from build123d import *

# Parameters (mm, degrees)
SKETCH1_R            = 4.5
SKETCH1_R_2          = 1.25
SKETCH1_R_3          = 1.75
SKETCH1_R_4          = 2.75
BOSS_EXTRUDE10_DEPTH = 5
SKETCH1_16_R         = 1.25
BOSS_EXTRUDE11_DEPTH = 5
SKETCH3_R            = 1.75
CUT_EXTRUDE5_DEPTH   = 17
CUT_EXTRUDE7_DEPTH   = 10
SKETCH1_18_R         = 4.5
SKETCH1_18_R_2       = 1.75
BOSS_EXTRUDE12_DEPTH = 5
SKETCH10_R           = 32.76798012
SKETCH10_R_2         = 29.85
BOSS_EXTRUDE13_DEPTH = 13
SKETCH11_R           = 27.095
CUT_EXTRUDE8_DEPTH   = 13
BOSS_EXTRUDE14_DEPTH = 3
SKETCH13_W           = 12
SKETCH13_H           = 4
BOSS_EXTRUDE15_DEPTH = 25
SKETCH14_R           = 1.25
CUT_EXTRUDE9_DEPTH   = 25
FILLET1_R            = 2.5
SKETCH18_W           = 172.850535033
SKETCH18_H           = 5
BOSS_EXTRUDE18_DEPTH = 18
SKETCH19_W           = 18
SKETCH19_H           = 172.850535033
BOSS_EXTRUDE19_DEPTH = 22
SKETCH20_R           = 7.5
CUT_EXTRUDE11_DEPTH  = 208
FILLET3_R            = 10


with BuildPart() as part:
    # Sketch1 → Boss-Extrude10 (new body)
    with BuildSketch(Plane(origin=(0, 0, 0), x_dir=(1, 0, 0), z_dir=(0, 1, 0))):
        with BuildLine():
            Line((-32.774, -22.380453712), (-32.774, 177.619546288))
            ThreePointArc((-32.774, 177.619546288), (0, 210.393546288), (32.774, 177.619546288))
            Line((32.774, 177.619546288), (32.774, -22.380453712))
            ThreePointArc((32.774, -22.380453712), (0, -55.154453712), (-32.774, -22.380453712))
        make_face()
        with Locations(Location((0, 177.619546288, 0), (0, 0, 270))):
            Circle(SKETCH1_R, mode=Mode.SUBTRACT)
        with Locations(Location((-6.733414, 37.119546288, 0), (0, 0, 270))):
            Circle(SKETCH1_R_2, mode=Mode.SUBTRACT)
        with Locations(Location((-6.733414, 27.619546288, 0), (0, 0, 270))):
            Circle(SKETCH1_R_2, mode=Mode.SUBTRACT)
        with Locations(Location((0, 53.605186475, 0), (0, 0, 270))):
            Circle(SKETCH1_R_3, mode=Mode.SUBTRACT)
        with Locations(Location((-14.032659813, 67.637846288, 0), (0, 0, 270))):
            Circle(SKETCH1_R_3, mode=Mode.SUBTRACT)
        with Locations(Location((0, 81.6705061, 0), (0, 0, 270))):
            Circle(SKETCH1_R_3, mode=Mode.SUBTRACT)
        with Locations(Location((14.032659813, 67.637846288, 0), (0, 0, 270))):
            Circle(SKETCH1_R_3, mode=Mode.SUBTRACT)
        with Locations(Location((0, 67.637846288, 0), (0, 0, 270))):
            Circle(SKETCH1_R, mode=Mode.SUBTRACT)
        with Locations(Location((0, -9.380453712, 0), (0, 0, 270))):
            Circle(SKETCH1_R_4, mode=Mode.SUBTRACT)
        with Locations(Location((11.258330249, -15.880453712, 0), (0, 0, 270))):
            Circle(SKETCH1_R_4, mode=Mode.SUBTRACT)
        with Locations(Location((11.258330249, -28.880453712, 0), (0, 0, 270))):
            Circle(SKETCH1_R_4, mode=Mode.SUBTRACT)
        with Locations(Location((0, -35.380453712, 0), (0, 0, 270))):
            Circle(SKETCH1_R_4, mode=Mode.SUBTRACT)
        with Locations(Location((-11.258330249, -28.880453712, 0), (0, 0, 270))):
            Circle(SKETCH1_R_4, mode=Mode.SUBTRACT)
        with Locations(Location((-11.258330249, -15.880453712, 0), (0, 0, 270))):
            Circle(SKETCH1_R_4, mode=Mode.SUBTRACT)
    extrude(amount=-BOSS_EXTRUDE10_DEPTH)

    # Sketch1_16 → Boss-Extrude11 (add)
    with BuildSketch(Plane(origin=(0, 0, 0), x_dir=(1, 0, 0), z_dir=(0, 1, 0))):
        with Locations((-6.733414, 37.119546288)):
            Circle(SKETCH1_16_R)
        with Locations((-6.733414, 27.619546288)):
            Circle(SKETCH1_16_R)
    extrude(amount=-BOSS_EXTRUDE11_DEPTH)

    # Sketch3 → Cut-Extrude5 (cut)
    with BuildSketch(Plane.XZ.offset(5)):
        with Locations(Location((15, -102.056321071, 0), (0, 0, 270))):
            Circle(SKETCH3_R)
        with Locations(Location((-30.384, -67.619546288, 0), (0, 0, 270))):
            Circle(SKETCH3_R)
        with Locations(Location((-30.384, -37.619546288, 0), (0, 0, 270))):
            Circle(SKETCH3_R)
        with Locations(Location((-30.384, -97.619546288, 0), (0, 0, 270))):
            Circle(SKETCH3_R)
        with Locations(Location((-30.384, -127.619546288, 0), (0, 0, 270))):
            Circle(SKETCH3_R)
        with Locations(Location((-30.384, -157.619546288, 0), (0, 0, 270))):
            Circle(SKETCH3_R)
        with Locations(Location((30.384, -157.619546288, 0), (0, 0, 90))):
            Circle(SKETCH3_R)
        with Locations(Location((30.384, -127.619546288, 0), (0, 0, 90))):
            Circle(SKETCH3_R)
        with Locations(Location((30.384, -97.619546288, 0), (0, 0, 90))):
            Circle(SKETCH3_R)
        with Locations(Location((30.384, -67.619546288, 0), (0, 0, 90))):
            Circle(SKETCH3_R)
        with Locations(Location((30.384, -37.619546288, 0), (0, 0, 90))):
            Circle(SKETCH3_R)
    extrude(amount=-CUT_EXTRUDE5_DEPTH, mode=Mode.SUBTRACT)

    # Sketch2 → Cut-Extrude7 (cut)
    with BuildSketch(Plane.XZ):
        with BuildLine():
            Line((28, 22.380453712), (28, -4.769011255))
            Line((28, -4.769011255), (32.774000001, -4.769011255))
            Line((32.774000001, -4.769011255), (32.774000001, 22.380453712))
            ThreePointArc((32.774000001, 22.380453712), (0, 55.154453713), (-32.774000001, 22.380453712))
            Line((-32.774000001, 22.380453712), (-32.774000001, -4.769011255))
            Line((-32.774000001, -4.769011255), (-28, -4.769011255))
            Line((-28, -4.769011255), (-28, 22.380453712))
            ThreePointArc((-28, 22.380453712), (0, 50.380453712), (28, 22.380453712))
        make_face()
        with BuildLine():
            Line((-28, -4.769011255), (28, -4.769011255))
            Line((28, -4.769011255), (28, 22.380453712))
            ThreePointArc((28, 22.380453712), (0, 50.380453712), (-28, 22.380453712))
            Line((-28, 22.380453712), (-28, -4.769011255))
        make_face()
    extrude(amount=CUT_EXTRUDE7_DEPTH, mode=Mode.SUBTRACT)

    # Sketch1_18 → Boss-Extrude12 (add)
    with BuildSketch(Plane(origin=(0, 0, 0), x_dir=(1, 0, 0), z_dir=(0, 1, 0))):
        with Locations((0, 67.637846288)):
            Circle(SKETCH1_18_R)
        with Locations((14.032659813, 67.637846288)):
            Circle(SKETCH1_18_R_2)
        with Locations((0, 81.6705061)):
            Circle(SKETCH1_18_R_2)
        with Locations((0, 53.605186475)):
            Circle(SKETCH1_18_R_2)
        with Locations((-14.032659813, 67.637846288)):
            Circle(SKETCH1_18_R_2)
    extrude(amount=-BOSS_EXTRUDE12_DEPTH)

    # Sketch10 → Boss-Extrude13 (add)
    with BuildSketch(Plane.XZ.offset(5)):
        with Locations(Location((0, -177.619546288, 0), (0, 0, 90))):
            Circle(SKETCH10_R)
        with Locations(Location((0, -177.619546288, 0), (0, 0, 90))):
            Circle(SKETCH10_R_2, mode=Mode.SUBTRACT)
    extrude(amount=BOSS_EXTRUDE13_DEPTH)

    # Sketch11 → Cut-Extrude8 (cut)
    with BuildSketch(Plane.XZ.offset(5)):
        with Locations(Location((0, -177.619546288, 0), (0, 0, 270))):
            Circle(SKETCH11_R)
    extrude(amount=-CUT_EXTRUDE8_DEPTH, mode=Mode.SUBTRACT)

    # Sketch5 → Boss-Extrude14 (add)
    with BuildSketch(Plane.XZ.offset(5)):
        Polygon((-7.824000001, -54.439091018), (-7.824000001, -50.294800153), (11.225999999, -50.294800153), (11.225999999, -52.737107845), (-5.625923078, -52.737107845), (-5.625923078, -55.667877076), align=None)
        Polygon((-7.824000001, -77.404415537), (-7.824000001, -74.946843422), (6.78786899, -68.867786932), (-7.824000001, -62.792546547), (-7.824000001, -60.308261691), (11.225999999, -68.478544143), (11.225999999, -69.260845826), align=None)
        Polygon((11.225999999, -103.048646307), (-7.824000001, -103.048646307), (-7.824000001, -102.144229239), (6.650489182, -90.592877076), (-7.824000001, -90.592877076), (-7.824000001, -88.150569384), (11.225999999, -88.150569384), (11.225999999, -89.150389095), (-3.210328126, -100.606338614), (11.225999999, -100.606338614), align=None)
        with BuildLine():
            Line((-7.824000001, -110.131338614), (-7.824000001, -107.689030922))
            Line((-7.824000001, -107.689030922), (4.963770432, -107.689030922))
            add(Edge.make_bspline(
                [(4.963770432, -107.689030922), (5.195284298, -107.690885051), (5.64058499, -107.694451338), (6.282127583, -107.710622767), (6.869902619, -107.750196634), (7.404321802, -107.799507581), (7.886610584, -107.856591103), (8.313879678, -107.93850968), (8.689949893, -108.026630447), (9.116491069, -108.169153007), (9.595339884, -108.393934907), (10.111712604, -108.751940741), (10.571673312, -109.196571131), (10.907530608, -109.628416016), (11.13794534, -110.012545465), (11.297510075, -110.317623544), (11.424793799, -110.643597173), (11.533834774, -110.983321068), (11.610882457, -111.340471014), (11.674764914, -111.711796449), (11.707736212, -112.10111909), (11.712193771, -112.36625392), (11.714461538, -112.501140297)],
                knots=[0, 0, 0, 0, 1.452629871, 2.794031722, 4.025694375, 5.147841271, 6.161522649, 7.070971626, 7.876222586, 8.582890533, 9.889534196, 11.180212824, 12.506716644, 13.889181747, 14.598189363, 15.315636514, 16.046279605, 16.790911698, 17.551832231, 18.336450274, 19.153675152, 20, 20, 20, 20], degree=3))
            add(Edge.make_bspline(
                [(11.714461538, -112.501140297), (11.709715065, -112.690996015), (11.700270364, -113.068777754), (11.611584234, -113.632488096), (11.470780234, -114.18810384), (11.271570837, -114.74809611), (10.996525721, -115.32564021), (10.608190367, -115.923011587), (10.131794371, -116.566713359), (9.758962639, -116.990402865), (9.562177884, -117.214030922)],
                knots=[0, 0, 0, 0, 0.856972921, 1.705235559, 2.570545082, 3.44278821, 4.385852251, 5.452194716, 6.655239899, 8, 8, 8, 8], degree=3))
            Line((9.562177884, -117.214030922), (7.80676923, -116.004325393))
            add(Edge.make_bspline(
                [(7.80676923, -116.004325393), (7.894907738, -115.863356861), (8.065044953, -115.59123978), (8.304537659, -115.195035974), (8.521847451, -114.828568699), (8.718040268, -114.494300424), (8.884251955, -114.186630498), (9.035266134, -113.914342494), (9.157620565, -113.667523035), (9.230416916, -113.512520303), (9.264521634, -113.439902316)],
                knots=[0, 0, 0, 0, 1.35182785, 2.609486248, 3.764263372, 4.816267098, 5.760612529, 6.607550145, 7.347644362, 8, 8, 8, 8], degree=3))
            add(Edge.make_bspline(
                [(9.264521634, -113.439902316), (9.30296182, -113.348904612), (9.376646938, -113.174473182), (9.457997196, -112.91437331), (9.506417053, -112.668323997), (9.513151386, -112.508961908), (9.516384615, -112.432450393)],
                knots=[0, 0, 0, 0, 1.132993667, 2.17180979, 3.122265503, 4, 4, 4, 4], degree=3))
            add(Edge.make_bspline(
                [(9.516384615, -112.432450393), (9.511267111, -112.318803952), (9.501130651, -112.093699551), (9.419283826, -111.764584671), (9.277522501, -111.45621453), (9.090739979, -111.16641845), (8.859379113, -110.901782723), (8.578900769, -110.678865607), (8.260942683, -110.493691853), (7.958995713, -110.380505827), (7.682179611, -110.302721603), (7.423123036, -110.262354362), (7.119487359, -110.218405126), (6.769344681, -110.184594649), (6.372022147, -110.164686683), (5.928147668, -110.144130246), (5.438290975, -110.133455838), (5.096065936, -110.13206328), (4.917977163, -110.131338614)],
                knots=[0, 0, 0, 0, 0.938055486, 1.858046901, 2.779836698, 3.729995872, 4.697713164, 5.669188152, 6.676648582, 7.724504959, 8.32352458, 9.04907482, 9.887175513, 10.858480013, 11.953077028, 13.173078688, 14.528912581, 16, 16, 16, 16], degree=3))
            Line((4.917977163, -110.131338614), (-7.824000001, -110.131338614))
        make_face()
    extrude(amount=BOSS_EXTRUDE14_DEPTH)

    # Sketch13 → Boss-Extrude15 (add)
    with BuildSketch(Plane.XZ.offset(5)):
        with Locations((0.000999999, -123.10114465)):
            Rectangle(SKETCH13_W, SKETCH13_H)
    extrude(amount=BOSS_EXTRUDE15_DEPTH)

    # Sketch14 → Cut-Extrude9 (cut)
    with BuildSketch(Plane(origin=(0, 0, -125.10114465), x_dir=(-1, 0, 0), z_dir=(0, 0, -1))):
        with Locations((0, -22.5)):
            Circle(SKETCH14_R)
        with Locations((0, -13)):
            Circle(SKETCH14_R)
    extrude(amount=-CUT_EXTRUDE9_DEPTH, mode=Mode.SUBTRACT)

    # Fillet1
    fillet1_edges = [part.edges().sort_by_distance(p)[0] for p in [
        (6.000999999, -5, -123.10114465),
        (-5.999000001, -5, -123.10114465),
        (6.000999999, -30, -123.10114465),
        (-5.999000001, -30, -123.10114465),
    ]]
    fillet(fillet1_edges, radius=FILLET1_R)

    # Sketch18 → Boss-Extrude18 (add)
    with BuildSketch(Plane(origin=(32.774, 0, 0), x_dir=(0, 0, -1), z_dir=(1, 0, 0))):
        with Locations((91.194278772, -2.5)):
            Rectangle(SKETCH18_W, SKETCH18_H)
    extrude(amount=BOSS_EXTRUDE18_DEPTH)

    # Sketch19 → Boss-Extrude19 (add)
    with BuildSketch(Plane(origin=(0, 0, 0), x_dir=(1, 0, 0), z_dir=(0, 1, 0))):
        with Locations((41.774, 91.194278772)):
            Rectangle(SKETCH19_W, SKETCH19_H)
    extrude(amount=BOSS_EXTRUDE19_DEPTH)

    # Sketch20 → Cut-Extrude11 (cut)
    with BuildSketch(Plane(origin=(0, 0, -177.619546288), x_dir=(-1, 0, 0), z_dir=(0, 0, -1))):
        with Locations((-41.774, 8.5)):
            Circle(SKETCH20_R)
    extrude(amount=-CUT_EXTRUDE11_DEPTH, mode=Mode.SUBTRACT)

    # Fillet3
    fillet3_edges = [part.edges().sort_by_distance(p)[0] for p in [
        (50.774, -5, -91.194278771),
        (50.774, 22, -91.194278771),
    ]]
    fillet(fillet3_edges, radius=FILLET3_R)


solid = part.part
The model under review builds one solid part; all positions refer to its coordinate system, in mm. A direction names the side the tool comes from. Give positions to 0.01 mm unless a question says otherwise; leave off trailing zeros. Order: outer loops, then holes, each group sorted by start corner. A loop starts at its lowest first (then second) coordinate and runs counter-clockwise, first axis right, second up. Notation, with made-up numbers: M 0,89.25 L 18,89.25 A19 ccw 18,99.25 Z; hole C -23.5,-3 d10. An arc over 180 degrees is marked long. Use one line per item in the form item = value. Start each with the question number.
Item 1: The part is to be moulded in two halves that separate along Z. For faces 1 (the flat face through (50.774, 8, -90)), 2 (the flat face through (34, 8, -177.62)), 3 (the cylindrical face through (-29.9, -2.5, -159.3)), say which applies: pulls with the +Z half, pulls with the -Z half, needs draft (parallel to the pull), parting line crosses it, or undercut.
Item 2: To check wall thickness, follow line 1 along Y through (x, z) = (0, -122); line 2 along Y through (x, z) = (-2.5, -124); line 3 along X through (y, z) = (-7, -170.5). State the ranges of each line that lie inside material, in increasing order. Write a range as from..to.
Item 3: We need section A-A on y = 8.5. Give the boundary of the cut face in (x, z).
Item 4: For faces 4 (the flat face through (0, -30, -123)), 5 (the flat face through (2.5, -8, -66.9)), 6 (the flat face through (0, 0, -83)), 7 (the cylindrical face through (30.307, -2.535, -129.368)), 8 (the flat face through (0, -17, -125.101)), list the 3-axis set-ups (+Z, -Z, +X, -X, +Y, -Y) from which the entire face can be reached by the end or side of a thin tool; tool diameter is ignored.
Item 5: Insertion check: pin 1 Ø4 at (x, z) = (30.38, -37.62) entering from +Y; pin 2 Ø3.5 at (x, y) = (1.5, -6) entering from -Z; pin 3 Ø1.2 at (y, z) = (-6.5, -101.5) entering from +X; pin 4 Ø4 at (x, y) = (1, -5.5) entering from +Z. Each pin has a flat end and moves straight along its axis. Give the tip position at first contact, or say it passes through.
Item 6: We need section B-B on x = 37. Give the boundary of the cut face in (y, z), plus the area to 3 significant figures.
Completed:
q1.face_1 = needs draft
q1.face_2 = pulls with the -Z half
q1.face_3 = undercut
q2.line_1 = -30..-23.75, -21.25..-14.25, -11.75..0
q2.line_2 = -30..0
q2.line_3 = -31.99..-28.99, 28.99..31.99
q3.outline = M 32.77,-177.62 L 34.27,-177.62 L 34.27,-4.77 L 32.77,-4.77 Z; M 49.27,-177.62 L 50.77,-177.62 L 50.77,-4.77 L 49.27,-4.77 Z
q4.face_4 = +Z, -Z, +X, -X, -Y
q4.face_5 = +Z, +X, -X, -Y
q4.face_6 = +Z, -Z, -X, +Y
q4.face_7 = +Y, -Y
q4.face_8 = +X, -X, -Y
q5.pin_1 = 0
q5.pin_2 = -210.39
q5.pin_3 = 11.23
q5.pin_4 = -4.77
q6.outline = M -5,-177.62 L 2.72,-177.62 L 2.72,-4.77 L -5,-4.77 Z; M 14.28,-177.62 L 22,-177.62 L 22,-4.77 L 14.28,-4.77 Z
q6.area = 2,670 mm²
